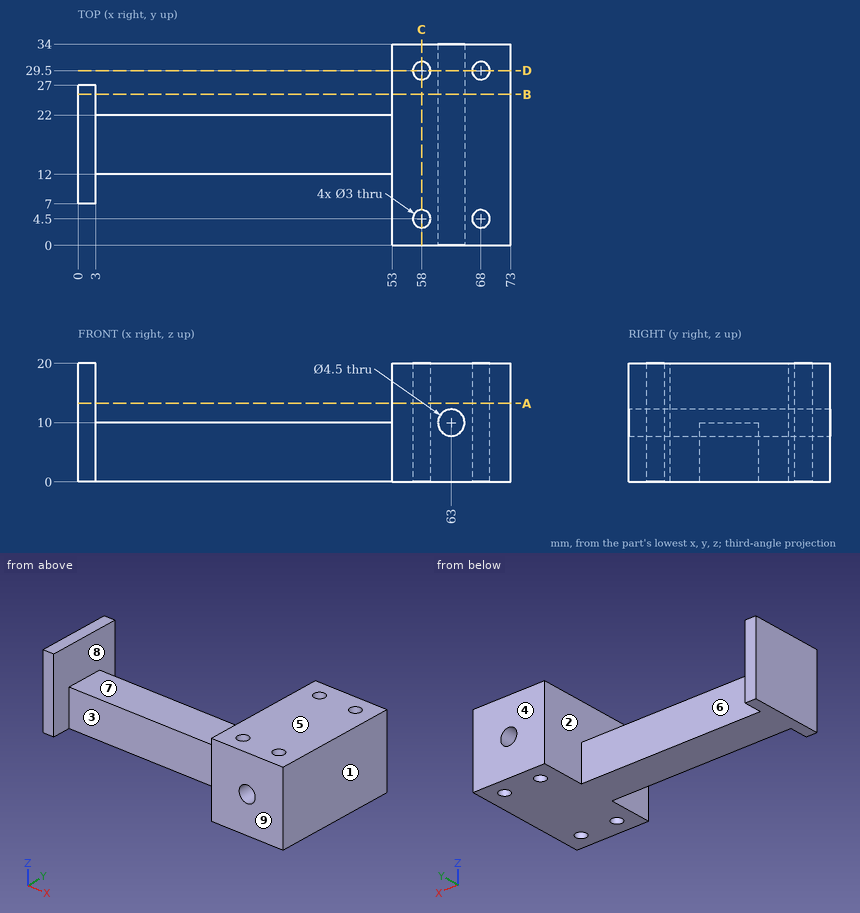
Print and shaded views of the part. All mm, measured from the part's lowest x, y and z. A direction names the side the tool comes from. Give positions to 0.01 mm unless a question says otherwise; leave off trailing zeros. Loops run counter-clockwise (first coordinate to the right, second up) from the corner with the lowest first, then second, coordinate; pieces in that order, holes last.
1) Pull direction X, two halves, no side cores. Call the marked faces 1, 2, 3 and 4: +X half, -X half, draft (parallel to the pull), parting line (faces both ways), or undercut.
2) Saw through at D-D (y = 29.5). Write the cut outline in (x, z).
3) Saw through at C-C (x = 58). Write the cut outline in (y, z).
4) Saw through at B-B (y = 25.5). Write the cut outline in (x, z), plus the area to 3 significant figures.
5) Tool access for the marked faces 5, 6, 7, 8 and 9: list every direction of +Z, -Z, +X, -X, +Y, -Y with a clear straight run to the whole face (end or side of a thin tool).
6) Saw through at A-A (z = 13.25). Write the cut outline in (x, y).
7) Flat gauge pins, fed straight in: pin 1 Ø2.5 at (x, y) = (58, 29.5) entering from -Z (3 decimals); pin 2 Ø1 at (x, z) = (25, 8.5) entering from -Y; pin 3 Ø3.5 at (x, z) = (2, 9) entering from -Y; pin 4 Ø2.5 at (x, z) = (1.5, 11) entering from +Y. Where does each tip first touch, or does it go through?
8) Wall check: line 1 (Y direction, x = 58, z = 6.75); line 2 (X direction, y = 4, z = 10.25); line 3 (Y direction, x = 59, z = 8.75). Give the ranges that are in metal, low to high.
Answer block:
1. face 1: +X half
1. face 2: undercut
1. face 3: undercut
1. face 4: draft
2. outline: (53, 0) - (56.5, 0) - (56.5, 20) - (53, 20) - close; (59.5, 0) - (66.5, 0) - (66.5, 20) - (59.5, 20) - close; (69.5, 0) - (73, 0) - (73, 20) - (69.5, 20) - close; hole circle Ø4.5 at (63, 10)
3. outline: (0, 0) - (3, 0) - (3, 20) - (0, 20) - close; (6, 0) - (28, 0) - (28, 20) - (6, 20) - close; (31, 0) - (34, 0) - (34, 20) - (31, 20) - close
4. outline: (0, 0) - (3, 0) - (3, 20) - (0, 20) - close; (53, 0) - (73, 0) - (73, 20) - (53, 20) - close; hole circle Ø4.5 at (63, 10)
4. area: 444 mm2
5. face 5: +Z, +X, -X, +Y, -Y
5. face 6: +Z, -Z, +Y
5. face 7: +Z, +Y, -Y
5. face 8: +Z
5. face 9: +Z, -Z, +X, -X, -Y
6. outline: (0, 7) - (3, 7) - (3, 27) - (0, 27) - close; (53, 0) - (73, 0) - (73, 34) - (53, 34) - close; hole circle Ø3 at (58, 4.5); hole circle Ø3 at (58, 29.5); hole circle Ø3 at (68, 4.5); hole circle Ø3 at (68, 29.5)
7. pin 1: passes through
7. pin 2: stops at y = 12
7. pin 3: stops at y = 7
7. pin 4: stops at y = 27
8. line 1: y = 0 to 3, 6 to 28, 31 to 34
8. line 2: x = 53 to 56.59, 59.41 to 60.76, 65.24 to 66.59, 69.41 to 73
8. line 3: y = 0 to 3.38, 5.62 to 28.38, 30.62 to 34
